```python
from build123d import *

# Parameters (mm, degrees)
SKETCH1_R           = 10
BOSS_EXTRUDE1_DEPTH = 50
BOSS_EXTRUDE2_DEPTH = 10
BOSS_EXTRUDE5_START = -25.31
SKETCH6_R           = 12.5
BOSS_EXTRUDE5_DEPTH = 5
LPATTERN1_COUNT     = 2
LPATTERN1_PITCH     = 15.25
CHAMFER2_SIZE       = 2.5
CUT_EXTRUDE1_START  = 10
SKETCH7_W           = 5
SKETCH7_H           = 5
CUT_EXTRUDE1_DEPTH  = 5
CHAMFER3_SIZE       = 1.5
SKETCH8_W           = 7.5
SKETCH8_H           = 7.5
BOSS_EXTRUDE6_DEPTH = 2
SKETCH10_R          = 10
SKETCH10_R_2        = 9.85
CUT_EXTRUDE3_DEPTH  = 10.25


with BuildPart() as part:
    # Sketch1 → Boss-Extrude1 (new body)
    with BuildSketch(Plane.XY):
        Circle(SKETCH1_R)
    extrude(amount=BOSS_EXTRUDE1_DEPTH)

    # Sketch2 → Boss-Extrude2 (add)
    with BuildSketch(Plane(origin=(0, 0, 0), x_dir=(-1, 0, 0), z_dir=(0, 0, -1))):
        with BuildLine():
            Line((-8.660254038, 5), (-13.660254038, 5))
            Line((-13.660254038, 5), (-13.660254038, -5))
            Line((-13.660254038, -5), (-8.660254038, -5))
            ThreePointArc((-8.660254038, -5), (-10, 0), (-8.660254038, 5))
        make_face()
        with BuildLine():
            Line((8.660254038, -5), (13.660254038, -5))
            Line((13.660254038, -5), (13.660254038, 5))
            Line((13.660254038, 5), (8.660254038, 5))
            ThreePointArc((8.660254038, 5), (10, 0), (8.660254038, -5))
        make_face()
    extrude(amount=-BOSS_EXTRUDE2_DEPTH)

    # Sketch6 → Boss-Extrude5 (add)
    with BuildSketch(Plane(origin=(0, 0, 0), x_dir=(-1, 0, 0), z_dir=(0, 0, -1)).offset(BOSS_EXTRUDE5_START)):
        Circle(SKETCH6_R)
    boss_extrude5 = extrude(amount=BOSS_EXTRUDE5_DEPTH)

    # LPattern1: Boss-Extrude5 ×2
    with Locations(*[(0, 0, i * LPATTERN1_PITCH) for i in range(1, LPATTERN1_COUNT)]):
        add(boss_extrude5)

    # Chamfer2
    chamfer2_edges = [part.edges().sort_by_distance(p)[0] for p in [
        (12.5, 0, 20.31),
        (12.5, 0, 40.56),
    ]]
    chamfer(chamfer2_edges, length=CHAMFER2_SIZE - 0.0001)  # a hair under: the kernel refuses the full size

    # Sketch7 → Cut-Extrude1 (cut)
    with BuildSketch(Plane(origin=(0, 0, 0), x_dir=(1, 0, 0), z_dir=(0, 1, 0)).offset(CUT_EXTRUDE1_START)):
        with Locations((0, -45.28)):
            Rectangle(SKETCH7_W, SKETCH7_H)
    extrude(amount=-CUT_EXTRUDE1_DEPTH, mode=Mode.SUBTRACT)

    # Chamfer3
    chamfer3_edges = [part.edges().sort_by_distance(p)[0] for p in [
        (2.5, 7.341229183, 47.78),
        (-2.5, 7.341229183, 47.78),
    ]]
    chamfer(chamfer3_edges, length=CHAMFER3_SIZE)

    # Sketch8 → Boss-Extrude6 (add)
    with BuildSketch(Plane.XY.offset(50)):
        Rectangle(SKETCH8_W, SKETCH8_H)
    extrude(amount=BOSS_EXTRUDE6_DEPTH)

    # Sketch10 → Cut-Extrude3 (cut)
    with BuildSketch(Plane.XY.offset(25.31)):
        with Locations(Location((0, 0, 0), (0, 0, 180))):
            Circle(SKETCH10_R)
        with Locations(Location((0, 0, 0), (0, 0, 180))):
            Circle(SKETCH10_R_2, mode=Mode.SUBTRACT)
    extrude(amount=CUT_EXTRUDE3_DEPTH, mode=Mode.SUBTRACT)


solid = part.part
```
The listing builds one solid part. Answer for the finished solid, in the listing's coordinates (mm). A direction names the side the tool comes from. Round coordinates to 2 decimals unless told otherwise and drop trailing zeros. Write each loop counter-clockwise with the first axis right and the second up, starting at its lowest first coordinate (ties: lowest second). Pieces come first, ordered by that corner, then holes. Notation, with made-up numbers: (-17.5, -19) -> (29.5, -19) arc R22 cw to (29.5, -6) -> close; hole circle Ø6 at (71.5, 63.25). An arc over 180 degrees is marked (long way). Use CSV: the item, a comma, the result in double quotes. Start each with the question number.
(1) The mould has two halves that part along Z. Classify faces 5 (the face through (0, 8, 47.78)), 6 (the face through (11, -5, 5)), 7 (the face through (2.19, -9.88, 40.44)), 8 (the face through (-2.5, 7, 45)): released by +Z, released by -Z, zero draft, split by the parting line, or undercut.
(2) Consider L1, parallel to Z at x = -6.5, y = 2.5; L2, parallel to Z at x = 12.5, y = 4.75; L3, parallel to X at y = 0, z = 10.5. Determine where each line is inside the solid, lowest interval first. Write a range as from..to.
(3) Which of the six approach directions +Z, -Z, +X, -X, +Y, -Y give full straight-line access (tool end or side, diameter ignored) to faces 1 (the face through (-11, 5, 5)), 2 (the face through (-11.923, 3.755, 24.077)), 3 (the face through (3.75, 0, 51)), 4 (the face through (-3.75, 0, 51))?
(4) Section D-D on z = 49 is taken. Give the vertices of the cut face in (x, y).
(5) Each of these flat-tipped pins is pushed along its axis until it touches: pin 1 (1.5 mm diameter, centred on x = 5.5, z = 41.5, fed in from +Y); pin 2 (5 mm diameter, centred on x = 10, z = 19, fed in from -Y); pin 3 (10 mm diameter, centred on x = 9, y = -6.5, fed in from +Z). Where does it stop, or does it pass through?
(6) Section B-B on z = 4.5 is taken. Give the vertices of the cut face in (x, y).
A:
1,face 5,"undercut"
1,face 6,"zero draft"
1,face 7,"released by +Z"
1,face 8,"undercut"
2,L1,"z = 0..50"
2,L2,"z = 0..10"
2,L3,"x = -10..10"
3,face 1,"-Z, -X, +Y"
3,face 2,"+Z"
3,face 3,"+Z, +X, +Y, -Y"
3,face 4,"+Z, -X, +Y, -Y"
4,outline,"circle Ø20 at (0, 0)"
5,pin 1,"stops at y = 8.8"
5,pin 2,"stops at y = -6.61"
5,pin 3,"stops at z = 50"
6,outline,"(-13.66, -5) -> (-8.66, -5) arc R10 ccw to (8.66, -5) -> (13.66, -5) -> (13.66, 5) -> (8.66, 5) arc R10 ccw to (-8.66, 5) -> (-13.66, 5) -> close"
